```python
from build123d import *

# Parameters (mm, degrees)
F1_DEPTH  = 25
F2_R      = 8.5
F3_DEPTH  = 25
F5_DEPTH  = 6
F6_W      = 28
F6_H      = 15
F7_DEPTH  = 6
F8_W      = 45
F8_H      = 30
F9_DEPTH  = 10
F11_DEPTH = 5
F13_W     = 45
F13_H     = 25
F14_DEPTH = 3
F15_DEPTH = 25
F16_W     = 45
F16_H     = 47
F17_DEPTH = 10
F19_DEPTH = 10


with BuildPart() as f1:
    # F0 (on Front) → F1 (new body)
    with BuildSketch(Plane.XZ):
        Polygon((13.583599414, 1.7193433519), (-9.416400586, 1.7193433519), (-3.6428978941, -8.2806566481), (-20.416400586, -8.2806566481), (-20.416400586, -58.2806566481), (24.583599414, -58.2806566481), (24.583599414, -8.2806566481), (7.8100967221, -8.2806566481), align=None)
    extrude(amount=F1_DEPTH)

    # F2 (on face) → F3 (cut)
    with BuildSketch(Plane.XZ.offset(25)):
        with Locations((2.083599414, -26.2928102165)):
            Circle(F2_R)
    extrude(amount=-F3_DEPTH, mode=Mode.SUBTRACT)

    # F4 (on face) → F5 (cut)
    with BuildSketch(Plane.XZ.offset(25)):
        with BuildLine():
            Line((11.083599414, -13.2806566481), (-6.916400586, -13.2806566481))
            ThreePointArc((-6.916400586, -13.2806566481), (-10.4519344919, -14.7451227421), (-11.916400586, -18.2806566481))
            Line((-11.916400586, -18.2806566481), (-11.916400586, -58.2806566481))
            Line((-11.916400586, -58.2806566481), (16.083599414, -58.2806566481))
            Line((16.083599414, -58.2806566481), (16.083599414, -18.2806566481))
            ThreePointArc((16.083599414, -18.2806566481), (14.6191333199, -14.7451227421), (11.083599414, -13.2806566481))
        make_face()
    extrude(amount=-F5_DEPTH, mode=Mode.SUBTRACT)

    # F6 (on face) → F7 (join)
    with BuildSketch(Plane.XZ.offset(19)):
        with Locations((2.083599414, -50.7806566481)):
            Rectangle(F6_W, F6_H)
    extrude(amount=F7_DEPTH)

    # F8 (on face) → F9 (join)
    with BuildSketch(Plane.XZ.offset(25)):
        Polygon((-11.916400586, -43.2806566481), (-20.416400586, -43.2806566481), (-20.416400586, -58.2806566481), (24.583599414, -58.2806566481), (24.583599414, -43.2806566481), (16.083599414, -43.2806566481), align=None)
        with Locations((2.083599414, -73.2806566481)):
            Rectangle(F8_W, F8_H)
    extrude(amount=F9_DEPTH)

    # F10 (on face) → F11 (cut)
    with BuildSketch(Plane.XZ.offset(35)):
        with BuildLine():
            Line((16.083599414, -43.2806566481), (-11.916400586, -43.2806566481))
            Line((-11.916400586, -43.2806566481), (-11.916400586, -76.2806566481))
            ThreePointArc((-11.916400586, -76.2806566481), (-10.4519344919, -79.816190554), (-6.916400586, -81.2806566481))
            Line((-6.916400586, -81.2806566481), (11.083599414, -81.2806566481))
            ThreePointArc((11.083599414, -81.2806566481), (14.6191333199, -79.816190554), (16.083599414, -76.2806566481))
            Line((16.083599414, -76.2806566481), (16.083599414, -43.2806566481))
        make_face()
    extrude(amount=-F11_DEPTH, mode=Mode.SUBTRACT)

    # F13 (on face) → F14 (cut)
    with BuildSketch(Plane(origin=(0, 0, -58.2806566481), x_dir=(1, 0, 0), z_dir=(0, 0, -1))):
        with Locations((2.083599414, 12.5)):
            Rectangle(F13_W, F13_H)
    extrude(amount=-F14_DEPTH, mode=Mode.SUBTRACT)

    # F12 (on face) → F15 (cut)
    with BuildSketch(Plane.XZ.offset(30)):
        with BuildLine():
            ThreePointArc((14.583599414, -62.2806566481), (13.1191333199, -58.7451227421), (9.583599414, -57.2806566481))
            Line((9.583599414, -57.2806566481), (-5.416400586, -57.2806566481))
            ThreePointArc((-5.416400586, -57.2806566481), (-8.9519344919, -58.7451227421), (-10.416400586, -62.2806566481))
            Line((-10.416400586, -62.2806566481), (-10.416400586, -74.2806566481))
            ThreePointArc((-10.416400586, -74.2806566481), (-8.9519344919, -77.816190554), (-5.416400586, -79.2806566481))
            Line((-5.416400586, -79.2806566481), (9.583599414, -79.2806566481))
            ThreePointArc((9.583599414, -79.2806566481), (13.1191333199, -77.816190554), (14.583599414, -74.2806566481))
            Line((14.583599414, -74.2806566481), (14.583599414, -62.2806566481))
        make_face()
    extrude(amount=-F15_DEPTH, mode=Mode.SUBTRACT)

    # F16 (on face) → F17 (cut)
    with BuildSketch(Plane(origin=(0, 0, 0), x_dir=(-1, 0, 0), z_dir=(0, 1, 0))):
        with Locations((-2.083599414, -31.7806566481)):
            Rectangle(F16_W, F16_H)
    extrude(amount=-F17_DEPTH, mode=Mode.SUBTRACT)

    # F18 (on face) → F19 (cut)
    with BuildSketch(Plane(origin=(0, 0, 0), x_dir=(-1, 0, 0), z_dir=(0, 1, 0))):
        Polygon((9.416400586, 1.7193433519), (-13.583599414, 1.7193433519), (-7.8100967221, -8.2806566481), (3.6428978941, -8.2806566481), align=None)
    extrude(amount=-F19_DEPTH, mode=Mode.SUBTRACT)


solid = f1.part
```
Model file for the job. Use its own axes, mm. A direction names the side the tool comes from. Coordinates: 2 decimals unless noted, no trailing zeros. Loops run counter-clockwise (first coordinate to the right, second up) from the corner with the lowest first, then second, coordinate; pieces in that order, holes last. Notation, with made-up numbers: (20, 89) -> (45, 89) arc R5 cw to (45, 94) -> close; hole circle Ø7 at (62.5, 10.5). An arc over 180 degrees is marked (long way). Answer as a JSON object with one key per item and string values.
Q1. Cut at A-A (y = -23.25). List the corners of the cut face in (x, z).
Report:
{"outline": "(-20.42, -55.28) -> (24.58, -55.28) -> (24.58, -8.28) -> (7.81, -8.28) -> (13.58, 1.72) -> (-9.42, 1.72) -> (-3.64, -8.28) -> (-20.42, -8.28) -> close; hole (-11.92, -43.28) -> (16.08, -43.28) -> (16.08, -18.28) arc R5 ccw to (11.08, -13.28) -> (-6.92, -13.28) arc R5 ccw to (-11.92, -18.28) -> close"}
Q2. Cut at D-D (z = -30). List the corners of the cut face in (x, y).
Report:
{"outline": "(-20.42, -25) -> (-11.92, -25) -> (-11.92, -19) -> (-5.57, -19) -> (-5.57, -10) -> (-20.42, -10) -> close; (9.73, -19) -> (16.08, -19) -> (16.08, -25) -> (24.58, -25) -> (24.58, -10) -> (9.73, -10) -> close"}
Q3. Cut at B-B (z = -63.5). List the corners of the cut face in (x, y), and give its area (3 significant figures).
Report:
{"outline": "(-20.42, -35) -> (-11.92, -35) -> (-11.92, -30) -> (-10.42, -30) -> (-10.42, -25) -> (-20.42, -25) -> close; (14.58, -30) -> (16.08, -30) -> (16.08, -35) -> (24.58, -35) -> (24.58, -25) -> (14.58, -25) -> close", "area": "185 mm2"}
Q4. 3-axis set-ups, long thin cutter, end or side, ignore diameter. For faces 1 (the flat face through (2, -25, -83)), 2 (the cylindrical face through (-8.913, -27.535, -58.706)), 3 (the flat face through (-11.916, -22, -31)), 4 (the flat face through (-11.916, -33, -60)): which of +Z, -Z, +X, -X, +Y, -Y reach the whole face in a straight line?
Report:
{"face 1": "-Z, +X, -X, +Y", "face 2": "+Y, -Y", "face 3": "-Y", "face 4": "+Z, -Y"}
Q5. Flat gauge pins, fed straight in: P1, Ø1, axis at x = 8, z = -37, coming from the -Y side; P2, Ø2.5, axis at x = 3.5, y = -28.5, coming from the +Z side; P3, Ø10, axis at x = 0, z = -11.5, coming from the -Y side. Where does each tip first touch, or does it go through?
Report:
{"P1": "stops at y = -19", "P2": "stops at z = -43.28", "P3": "stops at y = -25"}
Q6. Probe probe 1 along Z at (x, y) = (1.5, -22.25); probe 2 along X at (y, z) = (-22.75, -37); probe 3 along Z at (x, y) = (-5, -21). List the from-to ranges inside material, lowest first.
Report:
{"probe 1": "z = -55.28 to -43.28, -13.28 to 1.72", "probe 2": "x = -20.42 to -11.92, 16.08 to 24.58", "probe 3": "z = -55.28 to -43.28, -13.28 to -8.28, -5.93 to 1.72"}
Q7. Cut at C-C (x = 12.5). List the corners of the cut face in (y, z), and give its area (3 significant figures).
Report:
{"outline": "(-35, -88.28) -> (-25, -88.28) -> (-25, -78.34) -> (-30, -78.34) -> (-30, -81.08) -> (-35, -81.08) -> close; (-30, -58.22) -> (-25, -58.22) -> (-25, -55.28) -> (-10, -55.28) -> (-10, -8.28) -> (-25, -8.28) -> (-25, -13.49) -> (-19, -13.49) -> (-19, -43.28) -> (-30, -43.28) -> close; (-25, -0.16) -> (-10, -0.16) -> (-10, 1.72) -> (-25, 1.72) -> close", "area": "715 mm2"}
Q8. Pull direction Z, two halves, no side cores. Call faces 5 (the flat face through (2, -25, -10)), 6 (the flat face through (2, -30, -88.281)), 7 (the cylindrical face through (13.158, -27.535, -58.784)): released by +Z, released by -Z, zero draft, split by the parting line, or undercut.
Report:
{"face 5": "zero draft", "face 6": "released by -Z", "face 7": "undercut"}
